```python
from build123d import *

# Parameters (mm, degrees)
SALIENTE_EXTRUIR1_DEPTH = 10
CROQUIS2_R              = 2.5
CORTAR_EXTRUIR1_DEPTH   = 10
CROQUIS4_W              = 15
CROQUIS4_H              = 60
SALIENTE_EXTRUIR2_DEPTH = 15
SALIENTE_EXTRUIR3_DEPTH = 15
CROQUIS6_R              = 2.7
CORTAR_EXTRUIR2_DEPTH   = 15


with BuildPart() as part:
    # Croquis1 → Saliente-Extruir1 (new body)
    with BuildSketch(Plane.XY):
        Polygon((-7.5, 0), (-27.5, -35), (-7.5, -35), (11.843788115, -35), (31.843788115, -35), (7.5, 0), (7.5, 34.865095039), (-7.5, 34.865095039), align=None)
        Polygon((-10.268203217, -25), (0, -5), (12.707404341, -25), align=None, mode=Mode.SUBTRACT)
    extrude(amount=SALIENTE_EXTRUIR1_DEPTH)

    # Croquis2 → Cortar-Extruir1 (cut)
    with BuildSketch(Plane.XY.offset(10)):
        with Locations((0, 28.865095039)):
            Circle(CROQUIS2_R)
    extrude(amount=-CORTAR_EXTRUIR1_DEPTH, mode=Mode.SUBTRACT)

    # Croquis4 → Saliente-Extruir2 (add)
    with BuildSketch(Plane.XY.offset(10)):
        with Locations((0, 30)):
            Rectangle(CROQUIS4_W, CROQUIS4_H)
    extrude(amount=-SALIENTE_EXTRUIR2_DEPTH)

    # Croquis5 → Saliente-Extruir3 (add)
    with BuildSketch(Plane.XY.offset(10)):
        Polygon((-7.5, 0), (-27.5, -35), (31.843788115, -35), (7.5, 0), (-0.734678119, 11.839313291), align=None)
        Polygon((12.707404341, -25), (-10.268203217, -25), (0, -5), align=None, mode=Mode.SUBTRACT)
    extrude(amount=-SALIENTE_EXTRUIR3_DEPTH)

    # Croquis6 → Cortar-Extruir2 (cut)
    with BuildSketch(Plane.XY.offset(10)):
        with Locations((0, 55)):
            Circle(CROQUIS6_R)
    extrude(amount=-CORTAR_EXTRUIR2_DEPTH, mode=Mode.SUBTRACT)


solid = part.part
```
Geometry check sheet. Reference: the model listing, model coordinates, mm. A direction names the side the tool comes from. Round coordinates to 2 decimals unless told otherwise and drop trailing zeros. Write each loop counter-clockwise with the first axis right and the second up, starting at its lowest first coordinate (ties: lowest second). Pieces come first, ordered by that corner, then holes. Notation, with made-up numbers: (-6.75, -25.5) -> (19.25, -25.5) arc R18 cw to (19.25, 3.5) -> close; hole circle Ø1 at (15.25, 2.5). An arc over 180 degrees is marked (long way). Put each result on its own line as item: value.
1) Cross-section at A-A, the plane z = -4. Enter the section's corners in (x, y).
Recorded:
outline: (-27.5, -35) -> (31.84, -35) -> (7.5, 0) -> (7.5, 60) -> (-7.5, 60) -> (-7.5, 0) -> close; hole (-10.27, -25) -> (12.71, -25) -> (0, -5) -> close; hole circle Ø5.4 at (0, 55)
2) Cross-section at B-B, the plane y = 55. Enter the section's corners in (x, z).
Recorded:
outline: (-7.5, -5) -> (-2.7, -5) -> (-2.7, 10) -> (-7.5, 10) -> close; (2.7, -5) -> (7.5, -5) -> (7.5, 10) -> (2.7, 10) -> close
3) Cross-section at D-D, the plane x = 19. Enter the section's corners in (y, z), plus the area to 3 significant figures.
Recorded:
outline: (-35, -5) -> (-16.53, -5) -> (-16.53, 10) -> (-35, 10) -> close
area: 277 mm2
4) Access from +Z, -Z, +X, -X, +Y, -Y to the whole of each face (thin tool, end or side, straight path). Record for faces 4 (the face through (6.265, -14.86, 2.605)), 5 (the face through (0, 2, -5)), 6 (the face through (-7.5, 30, 3)), 7 (the face through (7.5, 30, 3)).
Recorded:
face 4: +Z, -Z
face 5: -Z, +X, -X, +Y, -Y
face 6: +Z, -Z, -X, +Y
face 7: +Z, -Z, +X, +Y
5) Thickness scan on probe 1 along X at (y, z) = (25.5, 2.5); probe 2 along Y at (x, z) = (-5, -2); probe 3 along X at (y, z) = (53, 2.5). Record the ranges inside material, lowest first. Write a range as from..to.
Recorded:
probe 1: x = -7.5..7.5
probe 2: y = -35..-25, -14.74..60
probe 3: x = -7.5..-1.81, 1.81..7.5
6) Release check for a two-part mould opening along X. For faces 1 (the face through (0, 60, 3)), 2 (the face through (-5.206, -15.14, 2.605)), 3 (the face through (-17.36, -17.255, 2.605)) record: pulls with the +X half, pulls with the -X half, needs draft (parallel to the pull), parting line crosses it, or undercut.
Recorded:
face 1: needs draft
face 2: undercut
face 3: pulls with the -X half
7) Depth check by flat-ended pin: P1, Ø6, axis at y = -3, z = 7.5, coming from the -X side; P2, Ø5, axis at y = 22, z = 2, coming from the -X side; P3, Ø3, axis at y = 27, z = 6.5, coming from the +X side. Enter the tip coordinate at first touch or a pass-through.
Recorded:
P1: stops at x = -10.93
P2: stops at x = -7.5
P3: stops at x = 7.5
8) Cross-section at C-C, the plane x = -4.5. Enter the section's corners in (y, z).
Recorded:
outline: (-35, -5) -> (-25, -5) -> (-25, 10) -> (-35, 10) -> close; (-13.76, -5) -> (60, -5) -> (60, 10) -> (-13.76, 10) -> close
